Part model, mm, in its own coordinate system. A direction names the side the tool comes from. Give positions to 0.01 mm unless a question says otherwise; leave off trailing zeros. Order: outer loops, then holes, each group sorted by start corner. A loop starts at its lowest first (then second) coordinate and runs counter-clockwise, first axis right, second up. Notation, with made-up numbers: M -13,86 L 23,86 A22 cw 23,123 Z; hole C 46.5,-36.75 d8. An arc over 180 degrees is marked long. Answer as a JSON object with one key per item and string values.
from build123d import *

# Parameters (mm, degrees)
PAD_DEPTH       = 3.5
PAD001_DEPTH    = 2
SKETCH002_R     = 1.7
POCKET_DEPTH    = 5
SKETCH003_W     = 23
SKETCH003_H     = 17
POCKET001_DEPTH = 5
SKETCH004_W     = 27.5
SKETCH004_H     = 28.2448
POCKET002_DEPTH = 1.5
PAD002_DEPTH    = 1.5
SKETCH006_R     = 2.5
POCKET003_DEPTH = 2


with BuildPart() as part:
    # Sketch → Pad (new body)
    with BuildSketch(Plane.XY):
        with BuildLine():
            Line((-37.5, 42.5), (37.5, 42.5))
            ThreePointArc((42.5, 37.5), (41.035534, 41.035534), (37.5, 42.5))
            Line((42.5, 37.5), (42.5, -37.5))
            ThreePointArc((37.5, -42.5), (41.035534, -41.035534), (42.5, -37.5))
            Line((37.5, -42.5), (-37.5, -42.5))
            ThreePointArc((-42.5, -37.5), (-41.035534, -41.035534), (-37.5, -42.5))
            Line((-42.5, -37.5), (-42.5, 37.5))
            ThreePointArc((-37.5, 42.5), (-41.035534, 41.035534), (-42.5, 37.5))
        make_face()
    extrude(amount=PAD_DEPTH)

    # Sketch001 (on Face10 of Pad) → Pad001 (join)
    with BuildSketch(Plane.XY.offset(3.5)):
        with BuildLine():
            Line((-30.5, 40.5), (30.5, 40.5))
            Line((30.5, 40.5), (30.5, 35.5))
            ThreePointArc((30.5, 35.5), (31.964466, 31.964466), (35.5, 30.5))
            Line((35.5, 30.5), (40.5, 30.5))
            Line((40.5, 30.5), (40.5, -30.5))
            Line((40.5, -30.5), (35.5, -30.5))
            ThreePointArc((35.5, -30.5), (31.964466, -31.964466), (30.5, -35.5))
            Line((30.5, -35.5), (30.5, -40.5))
            Line((30.5, -40.5), (-30.5, -40.5))
            Line((-30.5, -40.5), (-30.5, -35.5))
            ThreePointArc((-30.5, -35.5), (-31.964466, -31.964466), (-35.5, -30.5))
            Line((-35.5, -30.5), (-40.5, -30.5))
            Line((-40.5, -30.5), (-40.5, 30.5))
            Line((-40.5, 30.5), (-35.5, 30.5))
            ThreePointArc((-35.5, 30.5), (-31.964466, 31.964466), (-30.5, 35.5))
            Line((-30.5, 35.5), (-30.5, 40.5))
        make_face()
        with BuildLine():
            Line((-28.5, 38.5), (28.5, 38.5))
            Line((28.5, 38.5), (28.5, 35.5))
            ThreePointArc((28.5, 35.5), (30.550253, 30.550253), (35.5, 28.5))
            Line((35.5, 28.5), (38.5, 28.5))
            Line((38.5, 28.5), (38.5, -28.5))
            Line((38.5, -28.5), (35.5, -28.5))
            ThreePointArc((35.5, -28.5), (30.550253, -30.550253), (28.5, -35.5))
            Line((28.5, -35.5), (28.5, -38.5))
            Line((28.5, -38.5), (-28.5, -38.5))
            Line((-28.5, -38.5), (-28.5, -35.5))
            ThreePointArc((-28.5, -35.5), (-30.550253, -30.550253), (-35.5, -28.5))
            Line((-35.5, -28.5), (-38.5, -28.5))
            Line((-38.5, -28.5), (-38.5, 28.5))
            Line((-38.5, 28.5), (-35.5, 28.5))
            ThreePointArc((-35.5, 28.5), (-30.550253, 30.550253), (-28.5, 35.5))
            Line((-28.5, 35.5), (-28.5, 38.5))
        make_face(mode=Mode.SUBTRACT)
    extrude(amount=PAD001_DEPTH)

    # Sketch002 (on Face5 of Pad001) → Pocket (cut)
    with BuildSketch(Plane.XY.offset(3.5)):
        with Locations((-36.5, 36.5)):
            Circle(SKETCH002_R)
        with Locations((36.5, 36.5)):
            Circle(SKETCH002_R)
        with Locations((-36.5, -36.5)):
            Circle(SKETCH002_R)
        with Locations((36.5, -36.5)):
            Circle(SKETCH002_R)
    extrude(amount=-POCKET_DEPTH, mode=Mode.SUBTRACT)

    # Sketch003 (on Face48 of Pocket) → Pocket001 (cut)
    with BuildSketch(Plane.XY.offset(3.5)):
        Rectangle(SKETCH003_W, SKETCH003_H)
    extrude(amount=-POCKET001_DEPTH, mode=Mode.SUBTRACT)

    # Sketch004 (on Face35 of Pocket001) → Pocket002 (cut)
    with BuildSketch(Plane.XY.offset(3.5)):
        with Locations((0, -1.0224)):
            Rectangle(SKETCH004_W, SKETCH004_H)
    extrude(amount=-POCKET002_DEPTH, mode=Mode.SUBTRACT)

    # Sketch005 (on Face57 of Pocket002) → Pad002 (join)
    with BuildSketch(Plane.XY.offset(3.5)):
        Polygon((-15.25, 14.6), (-15.25, 9.1), (-13.75, 9.1), (-13.75, 13.1), (-9.75, 13.1), (-9.75, 14.6), align=None)
        Polygon((9.75, 13.1), (13.75, 13.1), (13.75, 9.1), (15.25, 9.1), (15.25, 14.6), (9.75, 14.6), align=None)
        Polygon((9.75, -15.1448), (13.75, -15.1448), (13.75, -11.1448), (15.25, -11.1448), (15.25, -16.6448), (9.75, -16.6448), align=None)
        Polygon((-13.75, -11.1448), (-13.75, -15.1448), (-9.75, -15.1448), (-9.75, -16.6448), (-15.25, -16.6448), (-15.25, -11.1448), align=None)
    extrude(amount=PAD002_DEPTH)

    # Sketch006 (on Face4 of Pad002) → Pocket003 (cut)
    with BuildSketch(Plane(origin=(0, 0, 0), x_dir=(1, 0, 0), z_dir=(0, 0, -1))):
        with Locations((-36.5, 36.5)):
            Circle(SKETCH006_R)
        with Locations((36.5, 36.5)):
            Circle(SKETCH006_R)
        with Locations((36.5, -36.5)):
            Circle(SKETCH006_R)
        with Locations((-36.5, -36.5)):
            Circle(SKETCH006_R)
    extrude(amount=-POCKET003_DEPTH, mode=Mode.SUBTRACT)


solid = part.part
1. Probe line 1 along X through (y, z) = (14, 4.1); line 2 along Y through (x, z) = (-36.5, 2.6); line 3 along Y through (x, z) = (-36.5, 1.45). List the from-to ranges inside material, lowest first.
Worked answers:
{"line 1": "x = -40.5 to -38.5, -15.25 to -9.75, 9.75 to 15.25, 38.5 to 40.5", "line 2": "y = -42.5 to -38.2, -34.8 to 34.8, 38.2 to 42.5", "line 3": "y = -42.5 to -39, -34 to 34, 39 to 42.5"}
2. Cut at B-B on y = -36.5. Give the cut face in (x, z).
Worked answers:
{"outline": "M -42.5,0 L -39,0 L -39,2 L -38.2,2 L -38.2,3.5 L -42.5,3.5 Z; M -34.8,2 L -34,2 L -34,0 L 34,0 L 34,2 L 34.8,2 L 34.8,3.5 L 30.5,3.5 L 30.5,5.5 L 28.5,5.5 L 28.5,3.5 L -28.5,3.5 L -28.5,5.5 L -30.5,5.5 L -30.5,3.5 L -34.8,3.5 Z; M 38.2,2 L 39,2 L 39,0 L 42.5,0 L 42.5,3.5 L 38.2,3.5 Z"}
3. Two-plate mould, pull along Y, no slides. Class faces 1 (the flat face through (-30.5, -38, 4)), 2 (the cylindrical face through (36.13, -38.16, 2.76)), 3 (the cylindrical face through (-41, 41.07, 1.73)): +Y half, -Y half, draft (parallel to the pull), parting line (faces both ways), or undercut.
Worked answers:
{"face 1": "draft", "face 2": "undercut", "face 3": "+Y half"}
4. Pin check, flat tips, straight feed: P1, Ø0.6, axis at x = -37, z = 5, coming from the -Y side; P2, Ø2, axis at y = -38.5, z = 5, coming from the -X side; P3, Ø1.2, axis at x = -11.5, z = 4.5, coming from the +Y side. Stop position of each tip, or through.
Worked answers:
{"P1": "stops at y = -30.5", "P2": "stops at x = -30.5", "P3": "stops at y = 40.5"}
5. Cut at A-A on x = 1. Give the cut face in (y, z).
Worked answers:
{"outline": "M -42.5,0 L -8.5,0 L -8.5,2 L -15.14,2 L -15.14,3.5 L -38.5,3.5 L -38.5,5.5 L -40.5,5.5 L -40.5,3.5 L -42.5,3.5 Z; M 8.5,0 L 42.5,0 L 42.5,3.5 L 40.5,3.5 L 40.5,5.5 L 38.5,5.5 L 38.5,3.5 L 13.1,3.5 L 13.1,2 L 8.5,2 Z"}
6. Which spindle directions (+Z, -Z, +X, -X, +Y, -Y) get a long thin tool onto all of the face, cutting with end or side? Do faces 4 (the flat face through (-30.5, 38, 4)), 5 (the cylindrical face through (30.6, -30.5, 4.5)), 6 (the flat face through (-11.5, 0, 1)), 7 (the flat face through (38, 30.5, 4)), 8 (the cylindrical face through (-34.19, -35.54, 0.99)). Say none if no direction does.
Worked answers:
{"face 4": "+Z, -X, +Y", "face 5": "+Z", "face 6": "+Z, -Z", "face 7": "+Z, +X, +Y", "face 8": "-Z"}
7. Cut at D-D on x = 21.5. Give the cut face in (y, z), plus the area to 4 significant figures.
Worked answers:
{"outline": "M -42.5,0 L 42.5,0 L 42.5,3.5 L 40.5,3.5 L 40.5,5.5 L 38.5,5.5 L 38.5,3.5 L -38.5,3.5 L -38.5,5.5 L -40.5,5.5 L -40.5,3.5 L -42.5,3.5 Z", "area": "305.5 mm^2"}
